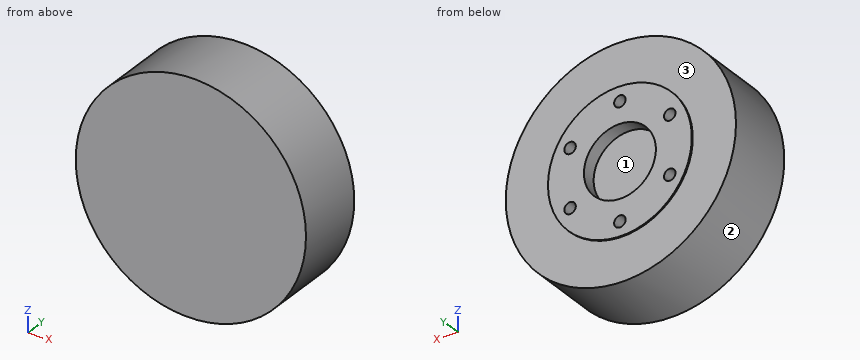
Autodesk Inventor part; units mm, degrees
ref_plane "XZ Plane" through (0, 0, 0) normal (0, 1, 0) x (-1, 0, 0)
ref_plane "XY Plane" through (0, 0, 0) normal (0, 0, 1) x (1, 0, 0)
sketch "Sketch1" plane through (0, 0, 0) normal (0, 1, 0) x (-1, 0, 0)
  circle A0 centre (0, 0) radius 80
  dimension "d0" = 160
extrude "Extrusion1" add sketch "Sketch1" along normal blind 50
sketch "Sketch2" plane through (0, 50, 0) normal (0, 1, 0) x (1, 0, 0)
  circle A0 centre (0, 0) radius 50
  dimension "d3" = 100
extrude "Extrusion2" add sketch "Sketch2" along normal blind 1
sketch "Sketch3" plane through (0, 51, 0) normal (0, 1, 0) x (1, 0, 0)
  circle A0 centre (0, 0) radius 25
  dimension "d6" = 50
extrude "Extrusion3" cut sketch "Sketch3" against normal blind 10
sketch "Sketch4" plane through (0, 51, 0) normal (0, 1, 0) x (1, 0, 0)
  circle A0 centre (0, 40) radius 4
  point P0 (0, 0)
  dimension "d9" = 8
  dimension "d10" = 40
extrude "Extrusion4" cut sketch "Sketch4" against normal blind 20
pattern_circular "Circular Pattern1" count 6 over 360 about axis through (0, 51, 0) along (0, -1, 0) of "Extrusion4"
properties part number "JR3_sensor"
Work out the finished part from the listing and answer in its coordinate system (mm). Face numbers are marked on the shaded views. Give positions to 0.01 mm unless a question says otherwise; leave off trailing zeros. Loops run counter-clockwise (first coordinate to the right, second up) from the corner with the lowest first, then second, coordinate; pieces in that order, holes last. Notation, with made-up numbers: (35.25, 24) -> (49.25, 24) arc R28 cw to (49.25, 54) -> close; hole circle Ø10 at (13, 10.25). An arc over 180 degrees is marked (long way). One line per question, with ' | ' between items. Start each with the question number.
1) Straight lines are drawn through the part: L1, parallel to Z at x = 0, y = 47; L2, parallel to Z at x = 0, y = 40.5; L3, parallel to X at y = 45, z = -22.5. For each, find the intervals that lie inside material, in ascending order.
2) Section D-D, the plane y = 35.5 is taken. Determine the outline of the cut face in (x, z), then the cut area to 3 significant figures.
3) Section C-C, the plane x = 0 is taken. Determine the outline of the cut face in (y, z).
4) Each of these flat-tipped pins is pushed along its axis until it touches: pin 1 (10 mm diameter, centred on x = 33.5, y = 39, fed in from -Z); pin 2 (1.5 mm diameter, centred on y = 26, z = -32.5, fed in from -X); pin 3 (4 mm diameter, centred on x = -0.5, z = -41.5, fed in from +Y). Where does it stop, or does it pass through?
5) Section B-B, the plane z = 0 is taken. Determine the outline of the cut face in (x, y), then the cut area to 3 significant figures.
6) Section A-A, the plane y = 44 is taken. Determine the outline of the cut face in (x, z).
7) Determine the mould class of the marked faces 1, 2 and 3 for opening direction X: +X half, -X half, draft (parallel to the pull), parting line (faces both ways), or undercut.
Resolved:
1) L1: -80 to -44, -36 to -25, 25 to 36, 44 to 80 | L2: -80 to -44, -36 to 36, 44 to 80 | L3: -76.77 to -37.76, -31.52 to -10.9, 10.9 to 31.52, 37.76 to 76.77
2) outline: circle Ø160 at (0, 0); hole circle Ø8 at (-34.64, -20); hole circle Ø8 at (-34.64, 20); hole circle Ø8 at (0, -40); hole circle Ø8 at (0, 40); hole circle Ø8 at (34.64, -20); hole circle Ø8 at (34.64, 20) | area: 19,800 mm2
3) outline: (0, -80) -> (50, -80) -> (50, -50) -> (51, -50) -> (51, -44) -> (31, -44) -> (31, -36) -> (51, -36) -> (51, -25) -> (41, -25) -> (41, 25) -> (51, 25) -> (51, 36) -> (31, 36) -> (31, 44) -> (51, 44) -> (51, 50) -> (50, 50) -> (50, 80) -> (0, 80) -> close
4) pin 1: z = -74.75 | pin 2: x = -73.43 | pin 3: y = 31
5) outline: (-80, 0) -> (80, 0) -> (80, 50) -> (50, 50) -> (50, 51) -> (25, 51) -> (25, 41) -> (-25, 41) -> (-25, 51) -> (-50, 51) -> (-50, 50) -> (-80, 50) -> close | area: 7,600 mm2
6) outline: circle Ø160 at (0, 0); hole circle Ø8 at (-34.64, -20); hole circle Ø8 at (-34.64, 20); hole circle Ø50 at (0, 0); hole circle Ø8 at (0, -40); hole circle Ø8 at (0, 40); hole circle Ø8 at (34.64, -20); hole circle Ø8 at (34.64, 20)
7) face 1: undercut | face 2: parting line | face 3: draft
